Design review of the part built by this model. Coordinates are the model's own, in mm. A direction names the side the tool comes from. Coordinates: 2 decimals unless noted, no trailing zeros. Loops run counter-clockwise (first coordinate to the right, second up) from the corner with the lowest first, then second, coordinate; pieces in that order, holes last. Notation, with made-up numbers: M 79.5,47.5 L 93.5,47.5 A25 ccw 93.5,60.5 Z; hole C 58,40.25 d2. An arc over 180 degrees is marked long. One line per item, written item: value.
```python
from build123d import *

# Parameters (mm, degrees)
F1_DEPTH = 12.7
F2_DEPTH = 0.508
F3_W     = 15.875
F3_H     = 4.7625
F4_DEPTH = 38.1
F5_W     = 9.388043
F5_H     = 4.7625
F5_W_2   = 6.856441
F5_H_2   = 9.525
F5_W_3   = 6.856442
F6_DEPTH = 14.478


with BuildPart() as f1:
    # F0 (on Front) → F1 (new body)
    with BuildSketch(Plane.XZ):
        Polygon((101.835918, 59.969447), (91.199405, 70.605959), (68.27643, 70.605959), (57.639918, 59.969447), (57.639918, 24.346472), (68.27643, 13.709959), (91.199405, 13.709959), (101.835918, 24.346472), align=None)
        Polygon((68.697271, 69.589959), (90.778564, 69.589959), (100.819918, 59.548606), (100.819918, 24.767313), (90.778564, 14.725959), (68.697271, 14.725959), (58.655918, 24.767313), (58.655918, 59.548606), align=None, mode=Mode.SUBTRACT)
        Polygon((100.819918, 59.548606), (90.778564, 69.589959), (68.697271, 69.589959), (58.655918, 59.548606), (58.655918, 24.767313), (68.697271, 14.725959), (90.778564, 14.725959), (100.819918, 24.767313), align=None)
        Polygon((69.538953, 67.557959), (89.936882, 67.557959), (98.787918, 58.706924), (98.787918, 25.608995), (89.936882, 16.757959), (69.538953, 16.757959), (60.687918, 25.608995), (60.687918, 58.706924), align=None, mode=Mode.SUBTRACT)
        Polygon((98.787918, 58.706924), (89.936882, 67.557959), (69.538953, 67.557959), (60.687918, 58.706924), (60.687918, 25.608995), (69.538953, 16.757959), (89.936882, 16.757959), (98.787918, 25.608995), align=None)
        Polygon((79.737918, 59.937959), (86.780575, 59.937959), (91.167918, 55.550616), (91.167918, 28.765302), (86.780575, 24.377959), (79.737918, 24.377959), (72.695261, 24.377959), (68.307918, 28.765302), (68.307918, 55.550616), (72.695261, 59.937959), align=None, mode=Mode.SUBTRACT)
        Polygon((79.737918, 57.905959), (79.737918, 59.937959), (72.695261, 59.937959), (68.307918, 55.550616), (68.307918, 28.765302), (72.695261, 24.377959), (79.737918, 24.377959), (79.737918, 26.409959), (73.536943, 26.409959), (70.339918, 29.606984), (70.339918, 54.708934), (73.536943, 57.905959), align=None)
        Polygon((79.737918, 56.889959), (79.737918, 57.905959), (73.536943, 57.905959), (70.339918, 54.708934), (70.339918, 29.606984), (73.536943, 26.409959), (79.737918, 26.409959), (79.737918, 27.425959), (73.957784, 27.425959), (71.355918, 30.027825), (71.355918, 54.288093), (73.957784, 56.889959), align=None)
        Polygon((85.938893, 57.905959), (79.737918, 57.905959), (79.737918, 56.889959), (85.518052, 56.889959), (88.119918, 54.288093), (88.119918, 30.027825), (85.518052, 27.425959), (79.737918, 27.425959), (79.737918, 26.409959), (85.938893, 26.409959), (89.135918, 29.606984), (89.135918, 54.708934), align=None)
        Polygon((91.167918, 55.550616), (86.780575, 59.937959), (79.737918, 59.937959), (79.737918, 57.905959), (85.938893, 57.905959), (89.135918, 54.708934), (89.135918, 29.606984), (85.938893, 26.409959), (79.737918, 26.409959), (79.737918, 24.377959), (86.780575, 24.377959), (91.167918, 28.765302), align=None)
    extrude(amount=-F1_DEPTH)

    # F0 (on Front) → F2 (cut)
    with BuildSketch(Plane.XZ):
        Polygon((100.819918, 59.548606), (90.778564, 69.589959), (68.697271, 69.589959), (58.655918, 59.548606), (58.655918, 24.767313), (68.697271, 14.725959), (90.778564, 14.725959), (100.819918, 24.767313), align=None)
        Polygon((69.538953, 67.557959), (89.936882, 67.557959), (98.787918, 58.706924), (98.787918, 25.608995), (89.936882, 16.757959), (69.538953, 16.757959), (60.687918, 25.608995), (60.687918, 58.706924), align=None, mode=Mode.SUBTRACT)
        Polygon((79.737918, 57.905959), (79.737918, 59.937959), (72.695261, 59.937959), (68.307918, 55.550616), (68.307918, 28.765302), (72.695261, 24.377959), (79.737918, 24.377959), (79.737918, 26.409959), (73.536943, 26.409959), (70.339918, 29.606984), (70.339918, 54.708934), (73.536943, 57.905959), align=None)
        Polygon((91.167918, 55.550616), (86.780575, 59.937959), (79.737918, 59.937959), (79.737918, 57.905959), (85.938893, 57.905959), (89.135918, 54.708934), (89.135918, 29.606984), (85.938893, 26.409959), (79.737918, 26.409959), (79.737918, 24.377959), (86.780575, 24.377959), (91.167918, 28.765302), align=None)
    extrude(amount=-F2_DEPTH, mode=Mode.SUBTRACT)

    # F3 (on face) → F4 (cut)
    with BuildSketch(Plane.XY.offset(70.605959)):
        with Locations((71.800418, 8.73125)):
            Rectangle(F3_W, F3_H)
        Polygon((95.612918, 11.1125), (79.737918, 11.1125), (79.737918, 6.35), (79.737918, 1.5875), (95.612918, 1.5875), align=None)
        with Locations((71.800418, 3.96875)):
            Rectangle(F3_W, F3_H)
    extrude(amount=-F4_DEPTH, mode=Mode.SUBTRACT)

    # F5 (on face) → F6 (cut)
    with BuildSketch(Plane(origin=(0, 0, 13.709959), x_dir=(1, 0, 0), z_dir=(0, 0, -1))):
        with Locations((75.043896, -3.96875)):
            Rectangle(F5_W, F5_H)
        with Locations((84.431939, -3.96875)):
            Rectangle(F5_W, F5_H)
        with Locations((75.043896, -8.73125)):
            Rectangle(F5_W, F5_H)
        with Locations((84.431939, -8.73125)):
            Rectangle(F5_W, F5_H)
        with Locations((62.940418, -6.35)):
            Rectangle(F5_W_2, F5_H_2)
        with Locations((96.535417, -6.35)):
            Rectangle(F5_W_3, F5_H_2)
    extrude(amount=-F6_DEPTH, mode=Mode.SUBTRACT)


solid = f1.part
```
(1) Tool access review of faces 1 (the flat face through (80, 1, 27.426)), 2 (the flat face through (72, 6, 28.188)), 3 (the flat face through (87.56, 0.25, 28.03)), 4 (the flat face through (80, 1.588, 60)): name each direction out of +Z, -Z, +X, -X, +Y, -Y from which nothing blocks a thin tool from reaching the whole face with its end or side.
Reply:
face 1: +Y, -Y
face 2: -Z
face 3: -Y
face 4: +Z
(2) We need section C-C on z = 62.5. State the section outline as (x, y) points.
Reply:
outline: M 60.17,0 L 61.61,0 L 61.61,0.51 L 64.48,0.51 L 64.48,0 L 94.99,0 L 94.99,0.51 L 97.87,0.51 L 97.87,0 L 99.31,0 L 99.31,12.7 L 60.17,12.7 Z; hole M 63.86,1.59 L 95.61,1.59 L 95.61,11.11 L 63.86,11.11 Z
(3) Insertion check: pin 1 (1 mm diameter, centred on y = 1.5, z = 61.5, fed in from -X); pin 2 (4 mm diameter, centred on x = 91, y = 6, fed in from +Z). Each pin has a flat end and moves straight along its axis. Give the tip position at first contact, or say it passes through.
Reply:
pin 1: stops at x = 58.67
pin 2: stops at z = 32.51
(4) We need section D-D on x = 97.5. State the section outline as (y, z) points, then the cut area to 3 significant figures.
Reply:
outline: M 0,20.01 L 1.59,20.01 L 1.59,28.19 L 11.11,28.19 L 11.11,20.01 L 12.7,20.01 L 12.7,64.31 L 0,64.31 L 0,62.87 L 0.51,62.87 L 0.51,59.99 L 0,59.99 L 0,24.32 L 0.51,24.32 L 0.51,21.45 L 0,21.45 Z
area: 482 mm2
(5) To check wall thickness, follow line 1 along X through (y, z) = (10, 27.5); line 2 along Y through (x, z) = (73, 20.5); line 3 along Y through (x, z) = (64.5, 63). State the ranges of each line that lie inside material, in increasing order. Write a range as [from, to].
Reply:
line 1: x = [57.64, 59.51], [66.37, 70.35], [89.13, 93.11], [99.96, 101.84]
line 2: y = [0, 1.59], [11.11, 12.7]
line 3: y = [0.51, 1.59], [11.11, 12.7]
(6) Mouldability with a two-part tool opening along Z and no side actions: class faces 5 (the flat face through (88, 6, 28.188)), 6 (the flat face through (96, 11.112, 23)), 7 (the flat face through (70.471, 0.25, 26.602)) as released by +Z, released by -Z, zero draft, split by the parting line, or undercut.
Reply:
face 5: released by -Z
face 6: zero draft
face 7: undercut
(7) We need section B-B on x = 76.5. State how many separate pieces and enclosed holes the cut face has, then the cut area to 3 significant figures.
Reply:
separate pieces: 4
enclosed holes: 0
area: 83.0 mm2
(8) We need section A-A on y = 10.5. State the section outline as (x, z) points.
Reply:
outline: M 57.64,24.35 L 59.51,22.47 L 59.51,28.19 L 66.37,28.19 L 66.37,15.62 L 68.28,13.71 L 70.35,13.71 L 70.35,28.19 L 73.2,28.19 L 71.36,30.03 L 71.36,32.51 L 63.86,32.51 L 63.86,66.19 L 57.64,59.97 Z; M 86.28,28.19 L 89.13,28.19 L 89.13,13.71 L 91.2,13.71 L 93.11,15.62 L 93.11,28.19 L 99.96,28.19 L 99.96,22.47 L 101.84,24.35 L 101.84,59.97 L 95.61,66.19 L 95.61,32.51 L 88.12,32.51 L 88.12,30.03 Z
